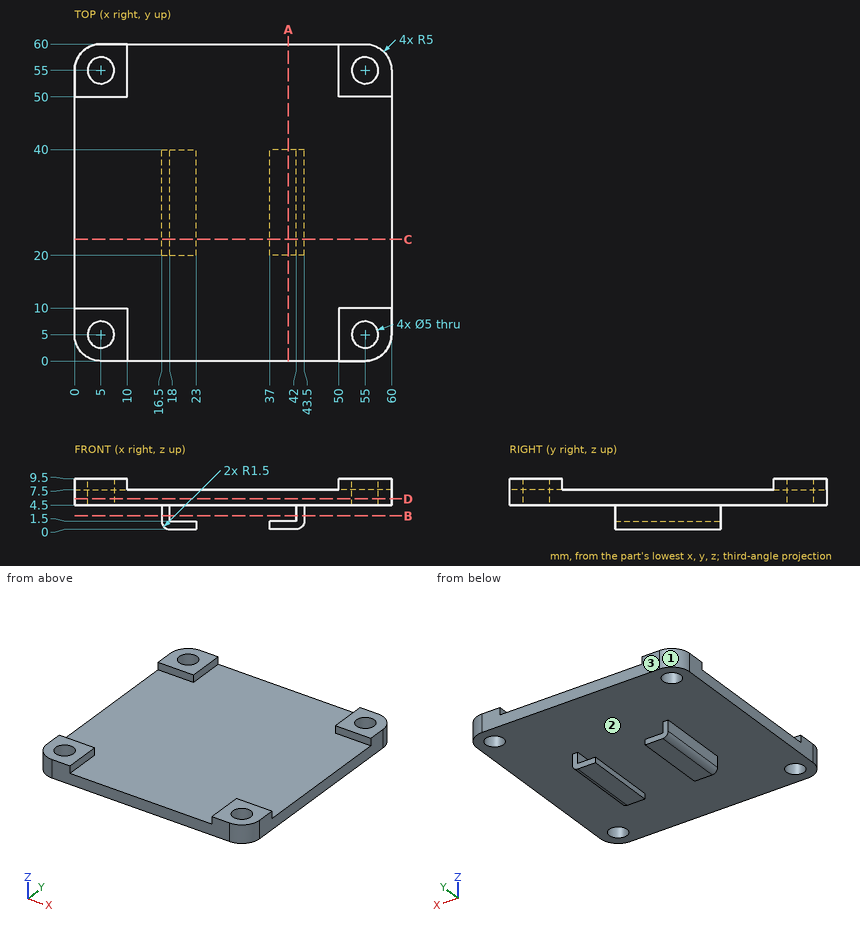
Study the drawing (mm; zero at the part's minimum x, y, z) and answer. Coordinates: 2 decimals unless noted, no trailing zeros. Loops run counter-clockwise (first coordinate to the right, second up) from the corner with the lowest first, then second, coordinate; pieces in that order, holes last. Notation, with made-up numbers: M 25.25,63.25 L 48.25,63.25 A20 ccw 48.25,86.25 Z; hole C 58,-6.5 d2. An arc over 180 degrees is marked long. Answer as a JSON object with one key per item and string values. Group by question number.
Item 1: Each of these flat-tipped pins is pushed along its axis until it touches: P1, Ø4, axis at x = 26, y = 29.5, coming from the +Z side; P2, Ø3.5, axis at x = 39.5, z = 2, coming from the +Y side; P3, Ø1.5, axis at x = 11.5, y = 53, coming from the -Z side. Where does it stop, or does it pass through?
Item 2: Section C-C (y = 23) is taken. Write down the section's boundary in (x, z), and give its area (3 significant figures).
Item 3: Section B-B (z = 2.5) is taken. Write down the section's boundary in (x, y), and give its area (3 significant figures).
Item 4: Consider L1, parallel to Y at x = 55, z = 6; L2, parallel to Y at x = 55, z = 8.2; L3, parallel to Y at x = 53, z = 8. Determine where each line is inside the solid, lowest interval first.
Item 5: Section A-A (x = 40.5) is taken. Write down the section's boundary in (y, z), and give its area (3 significant figures).
Item 6: Determine the mould class of the marked faces 1, 2 and 3 for opening direction X: +X half, -X half, draft (parallel to the pull), parting line (faces both ways), or undercut.
Item 7: Section D-D (z = 5.75) is taken. Write down the section's boundary in (x, y).
Solved:
{
 "1": {"P1": "stops at z = 7.5", "P2": "stops at y = 40", "P3": "stops at z = 4.5"},
 "2": {"outline": "M 0,4.5 L 16.5,4.5 L 16.5,1.5 A1.5 ccw 18,0 L 23,0 L 23,1.5 L 18,1.5 L 18,4.5 L 42,4.5 L 42,1.5 L 37,1.5 L 37,0 L 42,0 A1.5 ccw 43.5,1.5 L 43.5,4.5 L 60,4.5 L 60,7.5 L 0,7.5 Z", "area": "208 mm2"},
 "3": {"outline": "M 16.5,20 L 18,20 L 18,40 L 16.5,40 Z; M 42,20 L 43.5,20 L 43.5,40 L 42,40 Z", "area": "60.0 mm2"},
 "4": {"L1": "y = 0 to 2.5, 7.5 to 52.5, 57.5 to 60", "L2": "y = 0 to 2.5, 7.5 to 10, 50 to 52.5, 57.5 to 60", "L3": "y = 0 to 3.5, 6.5 to 10, 50 to 53.5, 56.5 to 60"},
 "5": {"outline": "M 0,4.5 L 60,4.5 L 60,7.5 L 0,7.5 Z; M 20,0 L 40,0 L 40,1.5 L 20,1.5 Z", "area": "210 mm2"},
 "6": {"face 1": "-X half", "face 2": "undercut", "face 3": "draft"},
 "7": {"outline": "M 0,5 A5 ccw 5,0 L 55,0 A5 ccw 60,5 L 60,55 A5 ccw 55,60 L 5,60 A5 ccw 0,55 Z; hole C 5,5 d5; hole C 5,55 d5; hole C 55,5 d5; hole C 55,55 d5"}
}
